Autodesk Inventor part; units mm, degrees
ref_plane "YZ Plane" through (0, 0, 0) normal (1, 0, 0) x (0, 1, 0)
ref_plane "XZ Plane" through (0, 0, 0) normal (0, 1, 0) x (-1, 0, 0)
ref_plane "XY Plane" through (0, 0, 0) normal (0, 0, 1) x (1, 0, 0)
sketch "Boceto1" plane through (0, 0, 0) normal (0, 0, 1) x (1, 0, 0)
  line L0 (0, 12) -> (0, 17.5)
  arc A0 (7, 24.5) -> (0, 17.5) centre (7, 17.5) ccw
  line L1 (7, 24.5) -> (15, 24.5)
  line L2 (15, 24.5) -> (15, 26.5)
  line L3 (0, 0) -> (11, 0)
  dimension "d0" = 49
  dimension "d1" = 15
  dimension "d2" = 2
  dimension "d3" = 7
  dimension "d4" = 12
surface revolve "SuperficieRevolución1" sketch "Boceto1" angle 360 about axis through (0, 0, 0) along (1, 0, 0) shown yes curves L2 L1 A0 L0
thicken "Engrosado1" operation new thickness 1 both sides no extend neighbours no toward (1, 0, 0) faces at (15, 25.5767, -2.114) (12.3333, 24.4206, -1.9714) (6.4769, 24.1634, -3.9269) (0, 15.4972, -1.396)
properties part number "cazoleta"
Check sheet for the modelled part. Datum: model origin and axes. Units: mm. A direction names the side the tool comes from. Give positions to 0.01 mm unless a question says otherwise; leave off trailing zeros. Loops run counter-clockwise (first coordinate to the right, second up) from the corner with the lowest first, then second, coordinate; pieces in that order, holes last. Notation, with made-up numbers: M 80,7.25 L 99,7.25 A34 ccw 99,46.25 Z; hole C 5,66.25 d8. An arc over 180 degrees is marked long. Use a Markdown table: item, result. Add a question column.
Q1. Sectioned sample at D-D, the plane x = 4.5. Record the cut outline in (y, z).
Q2. Scan lines: line 1 along Z through (x, y) = (13.25, 0); line 2 along Z through (x, y) = (13.25, -15.5); line 3 along Y through (x, z) = (15.25, 15). Record each from-to range of solid material in increasing order. Write a range as [from, to].
Q3. Mould release check, pull along Y, two halves, no side actions. Record for faces 4 (the flat face through (16, -16, -18)), 5 (the cylindrical face through (11.06, 13.17, 20.66)), 6 (the cylindrical face through (0.51, -11.99, 0.53)): pulls with the +Y half, pulls with the -Y half, needs draft (parallel to the pull), parting line crosses it, or undercut.
Q4. Go/stop test with flat-tipped pins: pin 1 (12 mm diameter, centred on y = -0.5, z = -5, fed in from +X); pin 2 (6 mm diameter, centred on y = 16.5, z = -8, fed in from +X); pin 3 (1 mm diameter, centred on x = 7.5, y = 1, fed in from +Z); pin 4 (4 mm diameter, centred on x = 6.5, z = 16.5, fed in from -Y). Record where each tip stops, or that it passes through.
Q5. Sectioned sample at A-A, the plane z = 0. Record the cut outline in (x, y).
Q6. Tool access check on faces 1 (the flat face through (15, 7.73, -23.43)), 2 (the flat face through (1, -12, -4)), 3 (the cylindrical face through (15.507, 14.246, 22.345)). Record the directions out of +Z, -Z, +X, -X, +Y, -Y that give a thin tool (end or side, any length) a straight path to the whole face; none if there is none.
Q7. Sectioned sample at C-C, the plane x = 10.5. Record the cut outline in (y, z), then the cut area to 3 significant figures.
Verdict:
| question | item | result |
|---|---|---|
| 1 | outline | C 0,0 d48.08; hole C 0,0 d45.91 |
| 2 | line 1 | [-24.5, -23.5], [23.5, 24.5] |
| 2 | line 2 | [-18.97, -17.66], [17.66, 18.97] |
| 2 | line 3 | [-21.85, -18.09], [18.09, 21.85] |
| 3 | face 4 | needs draft |
| 3 | face 5 | parting line crosses it |
| 3 | face 6 | undercut |
| 4 | pin 1 | through |
| 4 | pin 2 | x = 2.39 |
| 4 | pin 3 | z = 24.49 |
| 4 | pin 4 | y = -19.73 |
| 5 | outline | M 0,-17.5 A7 ccw 7,-24.5 L 15,-24.5 L 15,-26.5 L 16,-26.5 L 16,-23.5 L 7,-23.5 A6 cw 1,-17.5 L 1,-12 L 0,-12 Z; M 0,12 L 1,12 L 1,17.5 A6 cw 7,23.5 L 16,23.5 L 16,26.5 L 15,26.5 L 15,24.5 L 7,24.5 A7 ccw 0,17.5 Z |
| 6 | face 1 | -X |
| 6 | face 2 | +X |
| 6 | face 3 | +X, -X |
| 7 | outline | C 0,0 d49; hole C 0,0 d47 |
| 7 | area | 151 mm^2 |
